from build123d import *

# Parameters (mm, degrees)
BOSS_EXTRUDE1_DEPTH = 22
SKETCH2_W           = 5
SKETCH2_H           = 13
CUT_EXTRUDE1_DEPTH  = 10
SKETCH3_W           = 10
SKETCH3_H           = 4
SKETCH3_H_2         = 4.178443519
CUT_EXTRUDE2_DEPTH  = 5


with BuildPart() as part:
    # Sketch1 → Boss-Extrude1 (new body)
    with BuildSketch(Plane.XY):
        with BuildLine():
            Line((-61, 32), (61, 32))
            ThreePointArc((61, 32), (68.071067812, 29.071067812), (71, 22))
            Line((71, 22), (71, -22))
            ThreePointArc((71, -22), (68.071067812, -29.071067812), (61, -32))
            Line((61, -32), (-61, -32))
            ThreePointArc((-61, -32), (-68.071067812, -29.071067812), (-71, -22))
            Line((-71, -22), (-71, 22))
            ThreePointArc((-71, 22), (-68.071067812, 29.071067812), (-61, 32))
        make_face()
    extrude(amount=BOSS_EXTRUDE1_DEPTH)

    # Sketch2 → Cut-Extrude1 (cut)
    with BuildSketch(Plane.ZY.offset(71)):
        with Locations((15.5, 19.5)):
            Rectangle(SKETCH2_W, SKETCH2_H)
        with Locations((6.5, 19.5)):
            Rectangle(SKETCH2_W, SKETCH2_H)
    extrude(amount=-CUT_EXTRUDE1_DEPTH, mode=Mode.SUBTRACT)

    # Sketch3 → Cut-Extrude2 (cut)
    with BuildSketch(Plane(origin=(0, 32, 0), x_dir=(1, 0, 0), z_dir=(0, 1, 0))):
        with Locations((-25, -15)):
            Rectangle(SKETCH3_W, SKETCH3_H)
        with Locations((-45, -15.08922176)):
            Rectangle(SKETCH3_W, SKETCH3_H_2)
    extrude(amount=-CUT_EXTRUDE2_DEPTH, mode=Mode.SUBTRACT)


solid = part.part
Build history of the part. All positions in model axes, mm. A direction names the side the tool comes from. Coordinates: 2 decimals unless noted, no trailing zeros. Order: outer loops, then holes, each group sorted by start corner. A loop starts at its lowest first (then second) coordinate and runs counter-clockwise, first axis right, second up. Notation, with made-up numbers: (39.25, -19.75) - (43.25, -19.75) arc R15 ccw to (43.25, -1.75) - close; hole circle Ø7 at (25.5, 89.5). An arc over 180 degrees is marked (long way). Write each question's results on one line, items separated by ' | '. Start each with the question number.
Item 1: Band-saw the part on A-A on z = 15. Write the cut outline in (x, y).
Item 2: Mould opens along Z. For faces 1 (the face through (1, 0, 22)), 2 (the face through (-66, 13, 15)), 3 (the face through (1, 0, 0)) say: released by +Z, released by -Z, zero draft, split by the parting line, or undercut.
Item 3: Flat gauge pins, fed straight in: pin 1 (4.5 mm diameter, centred on y = 29.5, z = 15.5, fed in from +X); pin 2 (3.5 mm diameter, centred on y = 28.5, z = 15, fed in from -X); pin 3 (4 mm diameter, centred on x = -66.5, z = 6.5, fed in from -Y). Where does each tip first touch, or does it go through?
Item 4: Wall check: probe 1 along Y at (x, z) = (-62, 7.5); probe 2 along Y at (x, z) = (65, 7); probe 3 along X at (y, z) = (-27, 1). Give the ranges that are in metal, low to high. Write a range as [from, to].
Item 5: Band-saw the part on B-B on z = 7. Write the cut outline in (x, y).
Item 6: Tool access for faces 4 (the face through (-66, 19, 9)), 5 (the face through (-67.99, -29.15, 10.85)), 6 (the face through (-25, 27, 15)): list every direction of +Z, -Z, +X, -X, +Y, -Y with a clear straight run to the whole face (end or side of a thin tool).
Numbers:
1) outline: (-71, -22) arc R10 ccw to (-61, -32) - (61, -32) arc R10 ccw to (71, -22) - (71, 22) arc R10 ccw to (61, 32) - (-20, 32) - (-20, 27) - (-30, 27) - (-30, 32) - (-40, 32) - (-40, 27) - (-50, 27) - (-50, 32) - (-61, 32) arc R10 ccw to (-70.17, 26) - (-61, 26) - (-61, 13) - (-71, 13) - close
2) face 1: released by +Z | face 2: undercut | face 3: released by -Z
3) pin 1: x = 69.51 | pin 2: x = -69.8 | pin 3: y = -31.37
4) probe 1: [-31.95, 13], [26, 31.95] | probe 2: [-31.17, 31.17] | probe 3: [-69.66, 69.66]
5) outline: (-71, -22) arc R10 ccw to (-61, -32) - (61, -32) arc R10 ccw to (71, -22) - (71, 22) arc R10 ccw to (61, 32) - (-61, 32) arc R10 ccw to (-70.17, 26) - (-61, 26) - (-61, 13) - (-71, 13) - close
6) face 4: -X | face 5: +Z, -Z, -X, -Y | face 6: +Y
